For this review, use the dimensioned drawing (mm, ordinates from the lowest corner) and the shaded views. Round coordinates to 2 decimals unless told otherwise and drop trailing zeros. Loops run counter-clockwise (first coordinate to the right, second up) from the corner with the lowest first, then second, coordinate; pieces in that order, holes last. Notation, with made-up numbers: (-0.75, 26) -> (7.25, 26) arc R35 cw to (7.25, 64) -> close; hole circle Ø3 at (14, 67.5). An arc over 180 degrees is marked (long way). Answer as CSV lines item,"result". Start each with the question number.
(1) Take a section at C-C, the plane z = 4.8. Write out the cut boundary in (x, y), and give its area (3 significant figures).
(2) To check wall thickness, follow line 1 (Y direction, x = 16.75, z = 2.9); line 2 (Y direction, x = 28, z = 2.2) (1 decimal); line 3 (Z direction, x = 9.5, y = 2.3) (1 decimal). State the ranges of each line that lie inside material, in increasing order. Write a range as from..to.
(3) Take a section at A-A, the plane x = 12. Write out the cut boundary in (y, z).
(4) For P1, Ø2, axis at y = 0.5, z = 1.5, coming from the -X side; P2, Ø1.5, axis at x = 7, y = 2, coming from the +Z side, all flat-tipped, find the tip position at first contact; note any pin that passes through.
(5) Take a section at B-B, the plane y = 0.55. Write out the cut boundary in (x, z) (1 decimal), and give its area (3 significant figures).
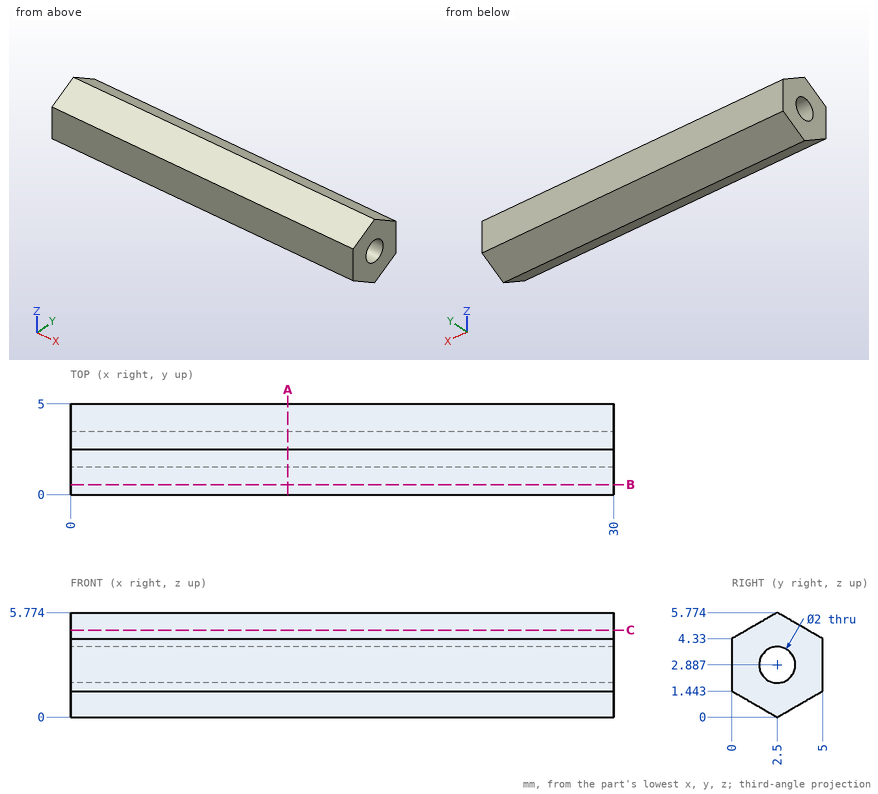
The answers:
1,outline,"(0, 0.81) -> (30, 0.81) -> (30, 4.19) -> (0, 4.19) -> close"
1,area,"101 mm²"
2,line 1,"0..1.5, 3.5..5"
2,line 2,"0..1.8, 3.2..5"
2,line 3,"0.1..1.9, 3.9..5.7"
3,outline,"(0, 1.44) -> (2.5, 0) -> (5, 1.44) -> (5, 4.33) -> (2.5, 5.77) -> (0, 4.33) -> close; hole circle Ø2 at (2.5, 2.89)"
4,P1,"x = 0"
4,P2,"z = 5.77"
5,outline,"(0, 1.1) -> (30, 1.1) -> (30, 4.6) -> (0, 4.6) -> close"
5,area,"106 mm²"
